Autodesk Inventor part; units mm, degrees
ref_plane "Work Plane1" through (0, 0, 10.287) normal (0, 0, -1) x (-1, 0, 0)
ref_plane "YZ Plane" through (0, 0, 0) normal (1, 0, 0) x (0, 1, 0)
ref_plane "XZ Plane" through (0, 0, 0) normal (0, 1, 0) x (-1, 0, 0)
sketch "Sketch1" plane through (0, 0, 0) normal (0, 0, 1) x (1, 0, 0)
  line L0 (0, 0) -> (38.1, 0)
  line L1 (38.1, 0) -> (38.1, 51.7633)
  line L2 (0, 86.36) -> (0, 0)
  line L3 (0, 86.36) -> (13.5942, 94.2086)
  line L4 (0, 86.36) -> (12.7, 64.363)
  line L5 (12.7, 64.363) -> (26.2942, 72.2116)
  line L6 (26.2942, 72.2116) -> (13.5942, 94.2086)
  line L7 (26.2942, 72.2116) -> (38.1, 51.7633)
  dimension "d0" = 15.6972
  dimension "d1" = 25.4
  dimension "d2" = 38.1
  dimension "d3" = 86.36
  dimension "d4" = 120
extrude "Extrusion1" add sketch "Sketch1" along normal blind 20.574 contours L2 L4 L5 L7 L1 L0
sketch "Sketch2" plane through (0, 0, 20.574) normal (0, 0, 1) x (1, 0, 0)
  line L0 (0, 86.36) -> (0, 0)
  line L1 (0, 0) -> (38.1, 0)
  line L2 (38.1, 0) -> (38.1, 51.7633)
  line L3 (38.1, 51.7633) -> (26.2942, 72.2116)
  line L4 (26.2942, 72.2116) -> (12.7, 64.363)
  line L5 (12.7, 64.363) -> (0, 86.36)
  line L6 (26.2942, 72.2116) -> (13.5942, 94.2086)
  line L7 (13.5942, 94.2086) -> (0, 86.36)
  line L8 (38.1, 51.7633) -> (26.2942, 72.2116)
extrude "Extrusion2" add sketch "Sketch2" along normal blind 2.54
ref_plane "Work Plane1" through (0, 0, 10.287) normal (0, 0, -1) x (-1, 0, 0)
mirror "Mirror1" about plane through (0, 0, 10.287) normal (0, 0, -1) of "Extrusion2"
sketch "Sketch3" plane through (0, 0, 23.114) normal (0, -1, 0) x (1, 0, 0)
  line L0 (38.1, -25.654) -> (38.1, 0)
  line L1 (38.1, -6.477) -> (33.02, -6.477)
  line L2 (33.02, -6.477) -> (33.02, -19.177)
  line L3 (33.02, -19.177) -> (38.1, -19.177)
  line L4 (38.1, -19.177) -> (38.1, -6.477)
  point P0 (0, -23.114)
  point P1 (38.1, -12.827)
  dimension "d9" = 12.7
  dimension "d10" = 6.35
  dimension "d11" = 5.08
extrude "Extrusion3" cut sketch "Sketch3" against normal blind 76.2
sketch "Sketch4" plane through (33.02, 0, 16.637) normal (1, 0, 0) x (0, 0, -1)
  circle A0 centre (6.35, 25.202) radius 1.778
  point P0 (16.637, 0)
extrude "Extrusion4" cut sketch "Sketch4" against normal blind 15.24
sketch "Sketch5" plane through (13.5942, 94.2086, 23.114) normal (0.8660254, 0.5, 0) x (0, 0, -1)
  line L0 (23.114, -25.4) -> (2.54, -25.4)
  line L1 (23.114, -25.4) -> (2.54, -25.4)
  line L2 (2.54, -25.4) -> (2.54, -37.7698)
  line L3 (2.54, -37.7698) -> (23.114, -37.7698)
  line L4 (23.114, -37.7698) -> (23.114, -25.4)
  point P0 (23.114, -74.79)
  dimension "d16" = 12.3698
extrude "Extrusion5" cut sketch "Sketch5" against normal blind 5.08
chamfer "Chamfer1" distance 1.016 angle 45 1 edges at (21.893, 69.6706, 10.287)
sketch "Sketch6" plane through (9.1948, 91.6686, 23.114) normal (0.8660254, 0.5, 0) x (0, 0, -1)
  line L0 (22.86, -25.4) -> (2.54, -25.4)
  line L1 (23.114, -37.7698) -> (2.54, -37.7698)
  circle A0 centre (12.827, -31.5849) radius 1.778
  line L2 (2.54, -37.7698) -> (2.54, 0)
  line L3 (2.54, -25.4) -> (2.54, -37.7698)
  point P0 (23.114, -74.79)
  point P1 (12.827, -37.7698)
  point P2 (2.54, -31.5849)
  dimension "d22" = 3.556
extrude "Extrusion6" cut sketch "Sketch6" against normal blind 7.62
ref_plane "Work Plane2" through (0, 0, 10.287) normal (0, 0, 1) x (1, 0, 0)
sketch "Sketch7" plane through (0, 0, 10.287) normal (0, 0, 1) x (1, 0, 0)
  line L0 (12.7, 64.363) -> (0, 86.36)
  line L1 (21.0149, 69.1636) -> (12.7, 64.363)
  line L2 (0, 0) -> (38.1, 0)
  line L3 (16.8574, 0) -> (11.3142, 0)
  line L4 (16.51, 66.5627) -> (11.43, 66.5627)
  line L5 (11.43, 66.5627) -> (11.43, 0)
  line L6 (11.43, 0) -> (16.51, 0)
  line L7 (16.51, 0) -> (16.51, 66.5627)
  dimension "d26" = 5.08
extrude "Extrusion7" cut sketch "Sketch7" along normal mid plane 10.16 contours L1 L7 L2 L5 L0
sketch "Sketch8" plane through (0, 0, 23.114) normal (-1, 0, 0) x (0, 0, 1)
  circle A0 centre (-12.827, 57.15) radius 1.778
  circle A1 centre (-12.827, 19.05) radius 1.778
  point P0 (-23.114, 0)
extrude "Extrusion8" cut sketch "Sketch8" against normal blind 15.24
sketch "Sketch9" plane through (0, 0, 23.114) normal (0, -1, 0) x (1, 0, 0)
  circle A0 centre (5.08, -12.827) radius 1.778
  circle A1 centre (22.86, -12.827) radius 1.778
  point P0 (0, -23.114)
extrude "Extrusion9" cut sketch "Sketch9" against normal blind 15.24
properties part number "PALM 3"
Geometry check sheet. Reference: the model listing, model coordinates, mm. A direction names the side the tool comes from. Give positions to 0.01 mm unless a question says otherwise; leave off trailing zeros. Write each loop counter-clockwise with the first axis right and the second up, starting at its lowest first coordinate (ties: lowest second). Pieces come first, ordered by that corner, then holes.
1) Section check D-D, the plane y = 8. Record the boundary of the cut face in (x, z).
2) Section check A-A, the plane z = 13.5. Record the boundary of the cut face in (x, y), and give its area (3 significant figures).
3) Access from +Z, -Z, +X, -X, +Y, -Y to the whole of each face (thin tool, end or side, straight path). Record for faces 1 (the cylindrical face through (25.5, 26.4, 11.6)), 2 (the flat face through (14, 34, 5.207)), 3 (the flat face through (36, 30, 3.937)).
4) Release check for a two-part mould opening along Y. For faces 4 (the flat face through (18.37, 60.53, 10.31)), 5 (the cylindrical face through (3.77, 7.51, 11.49)), 6 (the flat face through (6.7, 90.23, -1.25)) record: pulls with the +Y half, pulls with the -Y half, needs draft (parallel to the pull), parting line crosses it, or undercut.
5) Section check C-C, the plane x = 29. Record the boundary of the cut face in (y, z) (3 decimals).
6) Gauge pin test, flat ends, axial feed: pin 1 (1.1 mm diameter, centred on y = 24.5, z = 10.5, fed in from +X); pin 2 (5 mm diameter, centred on y = 73.5, z = 13.5, fed in from +X); pin 3 (3 mm diameter, centred on x = 22.86, z = 10.287, fed in from -Y). Record the tip position at first contact, or that the pin passes through.
7) Section check B-B, the plane y = 57.15. Record the boundary of the cut face in (x, z) (3 decimals).
8) Material ranges on L1, parallel to Z at x = 12.5, y = 29.5; L2, parallel to X at y = 24.5, z = 11; L3, parallel to Z at x = 34.5, y = 10, recorded low to high.
Computed:
1. outline: (0, -2.54) - (38.1, -2.54) - (38.1, 3.94) - (33.02, 3.94) - (33.02, 16.64) - (38.1, 16.64) - (38.1, 23.11) - (0, 23.11) - close; hole circle Ø3.56 at (5.08, 10.29); hole (11.43, 5.21) - (16.51, 5.21) - (16.51, 15.37) - (11.43, 15.37) - close; hole circle Ø3.56 at (22.86, 10.29)
2. outline: (0, 0) - (11.43, 0) - (11.43, 66.56) - (0, 86.36) - close; (16.51, 0) - (33.02, 0) - (33.02, 60.56) - (32.48, 61.5) - (28.08, 58.96) - (22.4, 68.79) - (21.01, 69.16) - (16.51, 66.56) - close
2. area: 1,940 mm2
3. face 1: +X
3. face 2: +Y, -Y
3. face 3: +X, +Y, -Y
4. face 4: undercut
4. face 5: needs draft
4. face 6: pulls with the +Y half
5. outline: (0, -2.54) - (67.525, -2.54) - (67.525, 0) - (59.49, 0) - (59.49, 20.574) - (67.525, 20.574) - (67.525, 23.114) - (0, 23.114) - close; hole circle Ø3.556 at (25.202, 10.287)
6. pin 1: stops at x = 17.78
6. pin 2: stops at x = 8.87
6. pin 3: stops at y = 15.24
7. outline: (0, -2.54) - (34.99, -2.54) - (34.99, 3.937) - (33.02, 3.937) - (33.02, 16.637) - (34.99, 16.637) - (34.99, 23.114) - (0, 23.114) - (0, 12.065) - (11.43, 12.065) - (11.43, 15.367) - (16.51, 15.367) - (16.51, 5.207) - (11.43, 5.207) - (11.43, 8.509) - (0, 8.509) - close
8. L1: z = -2.54 to 5.21, 15.37 to 23.11
8. L2: x = 0 to 11.43, 16.51 to 17.78
8. L3: z = -2.54 to 3.94, 16.64 to 23.11
